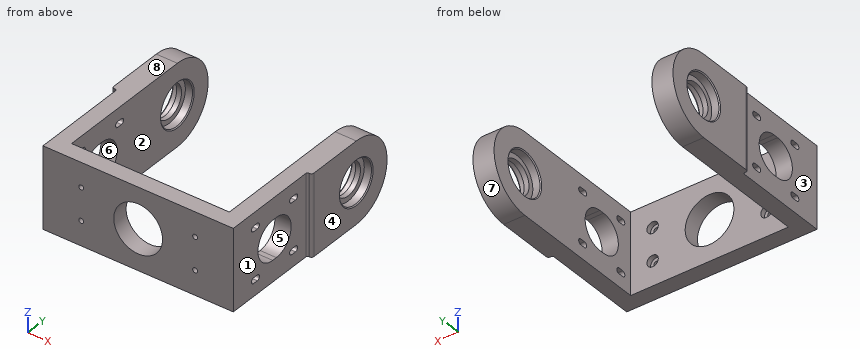
from build123d import *

# Parameters (mm, degrees)
BOSS_EXTRUDE1_DEPTH = 50
CUT_EXTRUDE1_DEPTH  = 121
SKETCH3_R           = 13.1
CUT_EXTRUDE2_DEPTH  = 5
CUT_EXTRUDE3_START  = -123
SKETCH3_3_R         = 13.1
CUT_EXTRUDE3_DEPTH  = 5
CUT_EXTRUDE4_START  = -13
SKETCH3_4_R         = 13.1
CUT_EXTRUDE4_DEPTH  = 5
CUT_EXTRUDE5_START  = -110
SKETCH3_5_R         = 13.1
CUT_EXTRUDE5_DEPTH  = 5
SKETCH4_R           = 10
CUT_EXTRUDE6_DEPTH  = 119
CHAMFER1_SIZE       = 0.6
CUT_EXTRUDE7_DEPTH  = 124
SKETCH7_R           = 15
CUT_EXTRUDE8_DEPTH  = 10
SKETCH6_R           = 1.5
CUT_EXTRUDE9_DEPTH  = 10
SKETCH8_R           = 3.5
CUT_EXTRUDE10_DEPTH = 3


with BuildPart() as part:
    # Sketch1 → Boss-Extrude1 (new body)
    with BuildSketch(Plane.XY):
        with BuildLine():
            Line((10, 128), (-3, 128))
            Line((-3, 128), (-3, 61.5))
            ThreePointArc((-3, 61.5), (-2.560660172, 60.439339828), (-1.5, 60))
            Line((-1.5, 60), (-1, 60))
            ThreePointArc((-1, 60), (-0.292893219, 59.707106781), (0, 59))
            Line((0, 59), (0, 0))
            Line((0, 0), (117, 0))
            Line((117, 0), (117, 59))
            ThreePointArc((117, 59), (117.292893219, 59.707106781), (118, 60))
            Line((118, 60), (118.5, 60))
            ThreePointArc((118.5, 60), (119.560660172, 60.439339828), (120, 61.5))
            Line((120, 61.5), (120, 128))
            Line((120, 128), (107, 128))
            Line((107, 128), (107, 10))
            Line((107, 10), (10, 10))
            Line((10, 10), (10, 128))
        make_face()
    extrude(amount=BOSS_EXTRUDE1_DEPTH)

    # Sketch2 → Cut-Extrude1 (cut, through all)
    with BuildSketch(Plane(origin=(117, 0, 0), x_dir=(0, 0, -1), z_dir=(1, 0, 0))):
        with BuildLine():
            Line((-42.25, 47.5), (-42.25, 50.5))
            ThreePointArc((-42.25, 50.5), (-40.5, 52.25), (-38.75, 50.5))
            Line((-38.75, 50.5), (-38.75, 47.5))
            ThreePointArc((-38.75, 47.5), (-40.5, 45.75), (-42.25, 47.5))
        make_face()
        with BuildLine():
            Line((-37, 35), (-37, 32))
            ThreePointArc((-37, 32), (-25, 20), (-13, 32))
            Line((-13, 32), (-13, 35))
            ThreePointArc((-13, 35), (-25, 47), (-37, 35))
        make_face()
        with BuildLine():
            Line((-11.25, 50.5), (-11.25, 47.5))
            ThreePointArc((-11.25, 47.5), (-9.5, 45.75), (-7.75, 47.5))
            Line((-7.75, 47.5), (-7.75, 50.5))
            ThreePointArc((-7.75, 50.5), (-9.5, 52.25), (-11.25, 50.5))
        make_face()
        with BuildLine():
            Line((-11.25, 19.5), (-11.25, 16.5))
            ThreePointArc((-11.25, 16.5), (-9.5, 14.75), (-7.75, 16.5))
            Line((-7.75, 16.5), (-7.75, 19.5))
            ThreePointArc((-7.75, 19.5), (-9.5, 21.25), (-11.25, 19.5))
        make_face()
        with BuildLine():
            Line((-38.75, 19.5), (-38.75, 16.5))
            ThreePointArc((-38.75, 16.5), (-40.5, 14.75), (-42.25, 16.5))
            Line((-42.25, 16.5), (-42.25, 19.5))
            ThreePointArc((-42.25, 19.5), (-40.5, 21.25), (-38.75, 19.5))
        make_face()
    extrude(amount=-CUT_EXTRUDE1_DEPTH, mode=Mode.SUBTRACT)

    # Sketch3 → Cut-Extrude2 (cut)
    with BuildSketch(Plane(origin=(120, 0, 0), x_dir=(0, 0, -1), z_dir=(1, 0, 0))):
        with Locations((-25, 96)):
            Circle(SKETCH3_R)
    extrude(amount=-CUT_EXTRUDE2_DEPTH, mode=Mode.SUBTRACT)

    # Sketch3<3> → Cut-Extrude3 (cut)
    with BuildSketch(Plane(origin=(120, 0, 0), x_dir=(0, 0, -1), z_dir=(1, 0, 0)).offset(CUT_EXTRUDE3_START)):
        with Locations((-25, 96)):
            Circle(SKETCH3_3_R)
    extrude(amount=CUT_EXTRUDE3_DEPTH, mode=Mode.SUBTRACT)

    # Sketch3<4> → Cut-Extrude4 (cut)
    with BuildSketch(Plane(origin=(120, 0, 0), x_dir=(0, 0, -1), z_dir=(1, 0, 0)).offset(CUT_EXTRUDE4_START)):
        with Locations((-25, 96)):
            Circle(SKETCH3_4_R)
    extrude(amount=CUT_EXTRUDE4_DEPTH, mode=Mode.SUBTRACT)

    # Sketch3<5> → Cut-Extrude5 (cut)
    with BuildSketch(Plane(origin=(120, 0, 0), x_dir=(0, 0, -1), z_dir=(1, 0, 0)).offset(CUT_EXTRUDE5_START)):
        with Locations((-25, 96)):
            Circle(SKETCH3_5_R)
    extrude(amount=-CUT_EXTRUDE5_DEPTH, mode=Mode.SUBTRACT)

    # Sketch4 → Cut-Extrude6 (cut, through all)
    with BuildSketch(Plane(origin=(115, 0, 0), x_dir=(0, 0, -1), z_dir=(1, 0, 0))):
        with Locations((-25, 96)):
            Circle(SKETCH4_R)
    extrude(amount=-CUT_EXTRUDE6_DEPTH, mode=Mode.SUBTRACT)

    # Chamfer1
    chamfer1_edges = [part.edges().sort_by_distance(p)[0] for p in [
        (120, 96, 38.1),
        (-3, 96, 38.1),
        (107, 96, 38.1),
        (10, 96, 38.1),
    ]]
    chamfer(chamfer1_edges, length=CHAMFER1_SIZE)

    # Sketch5 → Cut-Extrude7 (cut, through all)
    with BuildSketch(Plane.ZY.offset(3)):
        with BuildLine():
            Line((0, 96), (0, 151.710807056))
            Line((0, 151.710807056), (50, 151.710807056))
            Line((50, 151.710807056), (50, 96))
            ThreePointArc((50, 96), (25, 121), (0, 96))
        make_face()
    extrude(amount=-CUT_EXTRUDE7_DEPTH, mode=Mode.SUBTRACT)

    # Sketch7 → Cut-Extrude8 (cut)
    with BuildSketch(Plane(origin=(0, 10, 0), x_dir=(1, 0, 0), z_dir=(0, 1, 0))):
        with Locations((58.5, -25)):
            Circle(SKETCH7_R)
    extrude(amount=-CUT_EXTRUDE8_DEPTH, mode=Mode.SUBTRACT)

    # Sketch6 → Cut-Extrude9 (cut)
    with BuildSketch(Plane(origin=(0, 0, 0), x_dir=(-1, 0, 0), z_dir=(0, -1, 0))):
        with Locations((-93.5, -15)):
            Circle(SKETCH6_R)
        with Locations((-93.5, -35)):
            Circle(SKETCH6_R)
        with Locations((-23.5, -35)):
            Circle(SKETCH6_R)
        with Locations((-23.5, -15)):
            Circle(SKETCH6_R)
    extrude(amount=-CUT_EXTRUDE9_DEPTH, mode=Mode.SUBTRACT)

    # Sketch8 → Cut-Extrude10 (cut)
    with BuildSketch(Plane(origin=(0, 10, 0), x_dir=(1, 0, 0), z_dir=(0, 1, 0))):
        with Locations((23.5, -15)):
            Circle(SKETCH8_R)
        with Locations((23.5, -35)):
            Circle(SKETCH8_R)
        with Locations((93.5, -35)):
            Circle(SKETCH8_R)
        with Locations((93.5, -15)):
            Circle(SKETCH8_R)
    extrude(amount=-CUT_EXTRUDE10_DEPTH, mode=Mode.SUBTRACT)


solid = part.part
The model under review builds one solid part; all positions refer to its coordinate system, in mm. Face numbers are marked on the shaded views. A direction names the side the tool comes from. Coordinates: 2 decimals unless noted, no trailing zeros. Loops run counter-clockwise (first coordinate to the right, second up) from the corner with the lowest first, then second, coordinate; pieces in that order, holes last. Notation, with made-up numbers: M -34.75,-37.5 L 5.25,-37.5 A29 ccw 5.25,-11.5 Z; hole C 39,55.5 d9. An arc over 180 degrees is marked long. Put each result on its own line as item: value. Start each with the question number.
Q1. Add section C-C (y = 111.5). Write out the cut boundary in (x, z), and give its area (3 significant figures).
Q2. Add section A-A (x = 93.5). Write out the cut boundary in (y, z), and give its area (3 significant figures).
Q3. For the marked faces 1, 2, 3, 4 and 5, list the 3-axis set-ups (+Z, -Z, +X, -X, +Y, -Y) from which the entire face can be reached by the end or side of a thin tool; tool diameter is ignored.
Q4. Wall thickness on line 1 (Z direction, x = 23, y = 8); line 2 (X direction, y = 103, z = 33); line 3 (X direction, y = 4, z = 15): over which ranges is each line inside the solid? List them lowest first.
Q5. Clearance check with flat-ended pins moving along their axes: pin 1 (3.5 mm diameter, centred on x = 24, z = 33.5, fed in from +Y); pin 2 (2.5 mm diameter, centred on x = 93.5, z = 15, fed in from -Y); pin 3 (5 mm diameter, centred on x = 42, z = 39.5, fed in from +Y); pin 4 (25 mm diameter, centred on y = 43.5, z = 30, fed in from -X). State where each tip first meets the part, or that it passes through.
Q6. Add section D-D (z = 25). Count the separate pieces of the cut face and the enclosed holes in it, and give its area (3 significant figures).
Q7. The part is to be moulded in two halves that separate along Y. For the marked faces 6, 7 and 8, say which applies: +Y half, -Y half, draft (parallel to the pull), parting line (faces both ways), or undercut.
Q8. Add section B-B (x = 58.5). Write out the cut boundary in (y, z).
Answers:
1. outline: M -3,5.38 L 10,5.38 L 10,44.62 L -3,44.62 Z; M 107,5.38 L 120,5.38 L 120,44.62 L 107,44.62 Z
1. area: 1,020 mm^2
2. outline: M 0,0 L 10,0 L 10,11.5 L 7,11.5 L 7,13.5 L 0,13.5 Z; M 0,16.5 L 7,16.5 L 7,18.5 L 10,18.5 L 10,31.5 L 7,31.5 L 7,33.5 L 0,33.5 Z; M 0,36.5 L 7,36.5 L 7,38.5 L 10,38.5 L 10,50 L 0,50 Z
2. area: 416 mm^2
3. face 1: +Z, -Z, +X, -Y
3. face 2: +Z, -Z, +Y
3. face 3: +Z, -Z, -X, -Y
3. face 4: +Z, -Z, +X, +Y, -Y
3. face 5: +X, -X
4. line 1: z = 0 to 11.54, 18.46 to 31.54, 38.46 to 50
4. line 2: x = 2 to 5, 112 to 115
4. line 3: x = 0 to 22, 25 to 47.32, 69.68 to 92, 95 to 117
5. pin 1: stops at y = 7
5. pin 2: passes through
5. pin 3: stops at y = 10
5. pin 4: stops at x = 0
6. separate pieces: 6
6. enclosed holes: 0
6. area: 2,270 mm^2
7. face 6: undercut
7. face 7: +Y half
7. face 8: draft
8. outline: M 0,0 L 10,0 L 10,10 L 0,10 Z; M 0,40 L 10,40 L 10,50 L 0,50 Z
